For this review, take the finished solid that the model builds, in its own axes (mm). A direction names the side the tool comes from. Coordinates: 2 decimals unless noted, no trailing zeros. Loops run counter-clockwise (first coordinate to the right, second up) from the corner with the lowest first, then second, coordinate; pieces in that order, holes last.
```python
from build123d import *

# Parameters (mm, degrees)
SKETCH_1_R          = 3
EXTRUDE_1_DEPTH     = 5
SKETCH_3_R          = 1.5
CUT_EXTRUDE_1_DEPTH = 11


with BuildPart() as part:
    # 草圖1 → 填料-伸長1 (new body, symmetric)
    with BuildSketch(Plane(origin=(0, 0, 0), x_dir=(1, 0, 0), z_dir=(0, 1, 0))):
        Polygon((-55, -5), (-55, 0), (-45, 0), (-45, -5), (5, -5), (5, 5), (-57, 5), (-57, -5), align=None)
        Circle(SKETCH_1_R, mode=Mode.SUBTRACT)
    extrude(amount=EXTRUDE_1_DEPTH, both=True)

    # 草圖3 → 除料-伸長1 (cut, through all)
    with BuildSketch(Plane.XY.offset(5)):
        Circle(SKETCH_3_R)
    extrude(amount=-CUT_EXTRUDE_1_DEPTH, mode=Mode.SUBTRACT)


solid = part.part
```
Q1. Consider section B-B (y = -2.5). State the section outline as (x, z) points, then the cut area to 3 significant figures.
Q2. Consider section C-C (z = -1.5). State the section outline as (x, y) points.
Q3. For pin 1 Ø3 at (x, y) = (-47.5, -1) entering from +Z, flat-tipped, find the tip position at first contact; note if it passes through.
Q4. Consider section D-D (x = 0). State the section outline as (y, z) points, then the cut area to 3 significant figures.
Q5. Consider section A-A (z = 4.25). State the section outline as (x, y) points.
Q6. Machinability: for faces 1 (the face through (-26, -5, 0)), 2 (the face through (-55, 0, 3)), which of the approach directions +Z, -Z, +X, -X, +Y, -Y give a long, thin tool a straight path to every point of the face, cutting with its end or side? Answer none if there is none.
Q7. Wall thickness on probe 1 along X at (y, z) = (0, 3.25); probe 2 along X at (y, z) = (4.75, 2.75); probe 3 along X at (y, z) = (2.25, 4): over which ranges is each line inside the solid? List them lowest first.
Q8. The part is to be moulded in two halves that separate along X. For faces 3 (the face through (-50, 0, 0)), 4 (the face through (-56, 0, 5)), 5 (the face through (5, 0, 0)), say which applies: +X half, -X half, draft (parallel to the pull), parting line (faces both ways), or undercut.
Model answer:
1. outline: (-57, -5) - (5, -5) - (5, 5) - (-45, 5) - (-45, 0) - (-55, 0) - (-55, 5) - (-57, 5) - close; hole circle Ø6 at (0, 0)
1. area: 542 mm2
2. outline: (-57, -5) - (-2.6, -5) - (-2.6, 5) - (-57, 5) - close; (2.6, -5) - (5, -5) - (5, 5) - (2.6, 5) - close
3. pin 1: stops at z = 0
4. outline: (-5, -5) - (-1.5, -5) - (-1.5, -3) - (-5, -3) - close; (-5, 3) - (-1.5, 3) - (-1.5, 5) - (-5, 5) - close; (1.5, -5) - (5, -5) - (5, -3) - (1.5, -3) - close; (1.5, 3) - (5, 3) - (5, 5) - (1.5, 5) - close
4. area: 28.0 mm2
5. outline: (-57, -5) - (-55, -5) - (-55, 5) - (-57, 5) - close; (-45, -5) - (5, -5) - (5, 5) - (-45, 5) - close; hole circle Ø3 at (0, 0)
6. face 1: +Z, -Z, +X, -X, -Y
6. face 2: +Z, +Y, -Y
7. probe 1: x = -57 to -55, -45 to -1.5, 1.5 to 5
7. probe 2: x = -57 to -55, -45 to -1.2, 1.2 to 5
7. probe 3: x = -57 to -55, -45 to 5
8. face 3: undercut
8. face 4: draft
8. face 5: +X half
